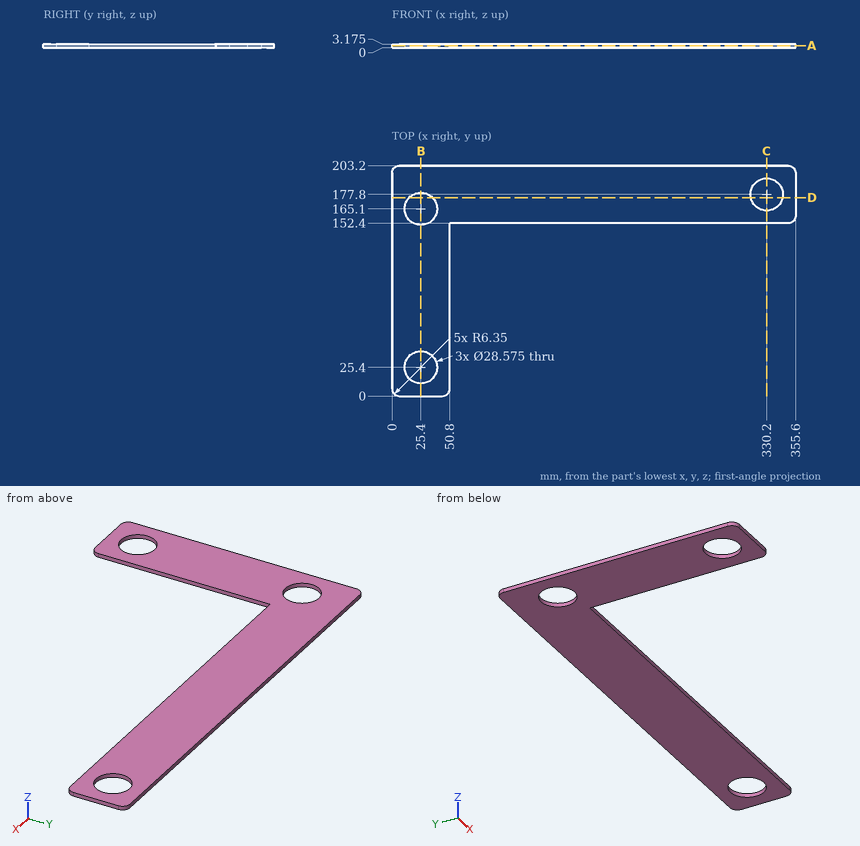
Here's the drawing with two shaded views (mm, measured from the low corner). I have some questions. Coordinates: 2 decimals unless noted, no trailing zeros. Order: outer loops, then holes, each group sorted by start corner. A loop starts at its lowest first (then second) coordinate and runs counter-clockwise, first axis right, second up.
Item 1: If we section it at A-A on z = 1.8: State how many separate pieces and enclosed holes the cut face has, plus the area to 3 significant figures.
Result sheet:
separate pieces: 1
enclosed holes: 3
area: 23,800 mm2
Item 2: I need wall thicknesses on line 1 (Y direction, x = 25.4, z = 1.5); line 2 (X direction, y = 165.1, z = 0.95); line 3 (Y direction, x = 22.5, z = 2.15). Which ranges of each line are inside material? Lowest first, please.
Result sheet:
line 1: y = 0 to 11.11, 39.69 to 150.81, 179.39 to 203.2
line 2: x = 0 to 11.11, 39.69 to 323.65, 336.75 to 355.6
line 3: y = 0 to 11.41, 39.39 to 151.11, 179.09 to 203.2
Item 3: If we section it at C-C on x = 330.2: List the corners of the cut face in (y, z) for me (1 decimal), plus the area to 3 significant figures.
Result sheet:
outline: (152.4, 0) - (163.5, 0) - (163.5, 3.2) - (152.4, 3.2) - close; (192.1, 0) - (203.2, 0) - (203.2, 3.2) - (192.1, 3.2) - close
area: 70.6 mm2
Item 4: If we section it at D-D on y = 175: List the corners of the cut face in (x, z) for me (3 decimals).
Result sheet:
outline: (0, 0) - (15.098, 0) - (15.098, 3.175) - (0, 3.175) - close; (35.702, 0) - (316.19, 0) - (316.19, 3.175) - (35.702, 3.175) - close; (344.21, 0) - (355.6, 0) - (355.6, 3.175) - (344.21, 3.175) - close
Item 5: If we section it at B-B on x = 25.4: List the corners of the cut face in (y, z) for me (1 decimal), plus the area to 3 significant figures.
Result sheet:
outline: (0, 0) - (11.1, 0) - (11.1, 3.2) - (0, 3.2) - close; (39.7, 0) - (150.8, 0) - (150.8, 3.2) - (39.7, 3.2) - close; (179.4, 0) - (203.2, 0) - (203.2, 3.2) - (179.4, 3.2) - close
area: 464 mm2
Item 6: For P1, Ø17, axis at x = 25.4, y = 165.1, coming from the +Z side, with a flat end and sliding along its axis, tell me the tip position at first contact or that it passes through.
Result sheet:
P1: passes through
